from build123d import *

# Parameters (mm, degrees)
F1_DEPTH = 10
F2_R     = 5
F4_DEPTH = 10.001


with BuildPart() as f1:
    # F0 (on Front) → F1 (new body)
    with BuildSketch(Plane.XZ):
        Polygon((-30, 100), (-50, 0), (50, 0), (30, 100), align=None)
    extrude(amount=F1_DEPTH)

    # F2
    f2_edges = [f1.edges().sort_by_distance(p)[0] for p in [
        (-30, -5, 100),
        (30, -5, 100),
        (-50, -5, 0),
        (50, -5, 0),
    ]]
    fillet(f2_edges, radius=F2_R)

    # F3 (on face) → F4 (cut, through all)
    with BuildSketch(Plane.XZ.offset(10)):
        Polygon((-16.890058, 72.688381), (-28.772679, 13.275276), (28.772679, 13.275276), (16.890058, 72.688381), align=None)
    extrude(amount=-F4_DEPTH, mode=Mode.SUBTRACT)


solid = f1.part
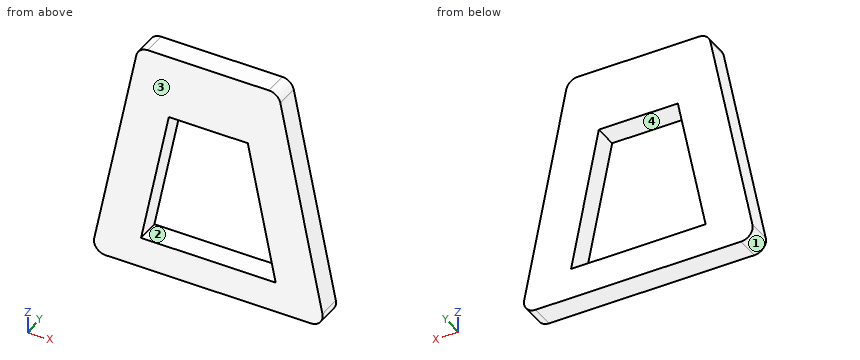
Input: part model. Units: mm. Frame: model coordinates. Face numbers are marked on the shaded views. Give positions to 0.01 mm unless a question says otherwise; leave off trailing zeros. Loops run counter-clockwise (first coordinate to the right, second up) from the corner with the lowest first, then second, coordinate; pieces in that order, holes last. Notation, with made-up numbers: (65.25, 50.25) -> (86.25, 50.25) arc R20 ccw to (86.25, 84.25) -> close; hole circle Ø9 at (32.25, 6.5). An arc over 180 degrees is marked (long way). Answer as a JSON object with one key per item and string values. Group by question number.
Item 1: Line query: probe 1 along Z at (x, y) = (-6.5, -7.5); probe 2 along X at (y, z) = (-8, 45); probe 3 along X at (y, z) = (-0.25, 51). Output: solid intervals per line, ascending.
Item 2: Cut plane C-C, the plane z = 55. Return the cut outline in (x, y).
Item 3: Cut plane D-D, the plane x = 42.5. Return the cut outline in (y, z), and give its area (3 significant figures).
Item 4: Pull-direction query (X, two-part tool) for the marked faces 1, 2, 3 and 4; classes: released by +X, released by -X, zero draft, split by the parting line, or undercut.
Item 5: Cut plane A-A, the plane y = -7.75. Return the cut outline in (x, z), and give its area (3 significant figures).
Item 6: Cut plane B-B, the plane x = 14.5. Return the cut outline in (y, z).
Checks:
{
 "1": {"probe 1": "z = 0 to 13.28, 72.69 to 100", "probe 2": "x = -41 to -22.43, 22.43 to 41", "probe 3": "x = -39.8 to -21.23, 21.23 to 39.8"},
 "2": {"outline": "(-39, -10) -> (-20.43, -10) -> (-20.43, 0) -> (-39, 0) -> close; (20.43, -10) -> (39, -10) -> (39, 0) -> (20.43, 0) -> close"},
 "3": {"outline": "(-10, 0) -> (0, 0) -> (0, 37.5) -> (-10, 37.5) -> close", "area": "375 mm²"},
 "4": {"face 1": "released by -X", "face 2": "undercut", "face 3": "zero draft", "face 4": "undercut"},
 "5": {"outline": "(-48.8, 5.98) arc R5 ccw to (-43.9, 0) -> (43.9, 0) arc R5 ccw to (48.8, 5.98) -> (30.8, 95.98) arc R5 ccw to (25.9, 100) -> (-25.9, 100) arc R5 ccw to (-30.8, 95.98) -> close; hole (-28.77, 13.28) -> (28.77, 13.28) -> (16.89, 72.69) -> (-16.89, 72.69) -> close", "area": "5,260 mm²"},
 "6": {"outline": "(-10, 0) -> (0, 0) -> (0, 13.28) -> (-10, 13.28) -> close; (-10, 72.69) -> (0, 72.69) -> (0, 100) -> (-10, 100) -> close"}
}
